Geometry: final body of the model. Coordinates: model frame, mm. Face numbers are marked on the shaded views. A direction names the side the tool comes from. Give positions to 0.01 mm unless a question says otherwise; leave off trailing zeros. Write each loop counter-clockwise with the first axis right and the second up, starting at its lowest first coordinate (ties: lowest second). Pieces come first, ordered by that corner, then holes.
Q1. Pin query (flat end, axial travel): pin 1 (6 mm diameter, centred on x = -40, z = -29.5, fed in from +Y); pin 2 (10 mm diameter, centred on y = 5.5, z = 18.5, fed in from -X) (3 decimals); pin 3 (1 mm diameter, centred on x = 4, y = 25.5, fed in from -Z) (3 decimals). Return the tip coordinate at first contact, or that it passes through.
Q2. Reachability of the marked faces 1 and 2 from +Z, -Z, +X, -X, +Y, -Y: full face, straight path, thin tool, end or side. Return the list, or none.
Q3. Cut plane D-D on x = -46. Return the cut outline in (y, z) (3 decimals), plus the area to 3 significant figures.
Q4. Line query: L1, parallel to Z at x = -40, y = 29 (3 decimals); L2, parallel to X at y = 29.35, z = 0 (3 decimals); L3, parallel to Z at x = 0, y = 28.35 (3 decimals). Output: solid intervals per line, ascending.
Q5. Cut plane A-A on y = 20.5. Return the cut outline in (x, z) (3 decimals).
Q6. Draft query along Z for the marked faces 3, 4 and 5. Return one class per face: pulls with the +Z half, pulls with the -Z half, needs draft (parallel to the pull), parting line crosses it, or undercut.
Autodesk Inventor part; units mm, degrees
ref_plane "YZ Plane" through (0, 0, 0) normal (1, 0, 0) x (0, 1, 0)
ref_plane "XZ Plane" through (0, 0, 0) normal (0, 1, 0) x (-1, 0, 0)
ref_plane "XY Plane" through (0, 0, 0) normal (0, 0, 1) x (1, 0, 0)
sketch "스케치2" plane through (0, 0, 0) normal (0, 1, 0) x (-1, 0, 0)
  line L0 (-49.375, 35.275) -> (49.375, 35.275)
  line L1 (49.375, 35.275) -> (49.375, -35.275)
  line L2 (49.375, -35.275) -> (-49.375, -35.275)
  line L3 (-49.375, -35.275) -> (-49.375, 35.275)
  line L4 (-49.375, 35.275) -> (49.375, -35.275) construction
  line L5 (49.375, 35.275) -> (-49.375, -35.275) construction
  line L6 (-54.375, -40.275) -> (54.375, -40.275)
  line L7 (54.375, -40.275) -> (54.375, 40.275)
  line L8 (54.375, 40.275) -> (-54.375, 40.275)
  line L9 (-54.375, 40.275) -> (-54.375, -40.275)
  point P0 (0, 0)
  dimension "d0" = 98.75
  dimension "d1" = 70.55
  dimension "d2" = 5
extrude "돌출1" add sketch "스케치2" along normal blind 32
sketch "스케치3" plane through (0, 0, 0) normal (0, 1, 0) x (-1, 0, 0)
  line L0 (-54.375, 40.275) -> (-54.375, -40.275) construction
  line L1 (54.375, -40.275) -> (-54.375, -40.275)
  line L2 (-54.375, -40.275) -> (-54.375, 40.275)
  line L3 (-54.375, 40.275) -> (54.375, 40.275)
  line L4 (54.375, 40.275) -> (54.375, -40.275)
  line L5 (54.375, -40.275) -> (-54.375, 40.275) construction
  line L6 (-54.375, -40.275) -> (54.375, 40.275) construction
  point P0 (0, 0)
extrude "돌출2" add sketch "스케치3" against normal blind 5
sketch "스케치4" plane through (0, 0, 0) normal (0, 1, 0) x (-1, 0, 0)
  line L0 (49.375, 35.275) -> (49.375, -35.275) construction
  line L1 (54.375, -40.275) -> (54.375, 40.275) construction
  line L2 (49.375, 30.275) -> (54.375, 30.275)
  line L3 (54.375, 30.275) -> (54.375, -30.275)
  line L4 (54.375, -30.275) -> (49.375, -30.275)
  line L5 (49.375, -30.275) -> (49.375, 30.275)
  line L6 (-49.375, 35.275) -> (49.375, 35.275) construction
  line L7 (49.375, -35.275) -> (-49.375, -35.275) construction
  line L8 (54.375, -40.275) -> (-54.375, -40.275) construction
  line L9 (-44.375, -35.275) -> (14.375, -35.275)
  line L10 (14.375, -35.275) -> (14.375, -40.275)
  line L11 (14.375, -40.275) -> (-44.375, -40.275)
  line L12 (-44.375, -40.275) -> (-44.375, -35.275)
  line L13 (-49.375, -35.275) -> (-49.375, 35.275) construction
  point P0 (0, 0)
  dimension "d7" = 5
  dimension "d8" = 5
  dimension "d11" = 5
  dimension "d12" = 35
extrude "돌출3" cut sketch "스케치4" along normal through all
sketch "스케치5" plane through (0, 32, 0) normal (0, 1, 0) x (1, 0, 0)
  line L0 (49.375, 35.275) -> (49.375, -35.275) construction
  line L1 (49.375, -35.275) -> (-49.375, -35.275) construction
  circle A0 centre (0, -37.775) radius 1.5
  circle A1 centre (51.875, 0) radius 1.5
  circle A2 centre (-34.375, 37.775) radius 1.5
  line L2 (-49.375, 35.275) -> (-14.375, 35.275) construction
  line L3 (-54.375, 40.275) -> (-54.375, 30.275) construction
  point P0 (0, 0)
  dimension "d17" = 3
  dimension "d18" = 2.5
  dimension "d19" = 3
  dimension "d20" = 2.5
  dimension "d21" = 3
  dimension "d22" = 2.5
  dimension "d23" = 20
extrude "돌출4" cut sketch "스케치5" against normal blind 5
fillet "모깎기1" radius 2.5 14 edges at (-54.375, 13.5, 40.275) (54.375, 13.5, 40.275) (54.375, 13.5, -40.275) (-54.375, 13.5, -40.275) (-54.375, -5, 0) (0, -5, -40.275) (0, -5, 40.275) (54.375, -5, 0) (-14.375, 16, -40.275) (15, 0, -40.275) (44.375, 16, -40.275) (-54.375, 16, 30.275) (-54.375, 0, 0) (-54.375, 16, -30.275)
chamfer "모따기1" distance 2 angle 45 6 edges at (-31.875, 32, -35.275) (-49.375, 32, -32.775) (-49.375, 32, 32.775) (0, 32, 35.275) (49.375, 32, 0) (46.875, 32, -35.275)
properties part number "housing_bottom"
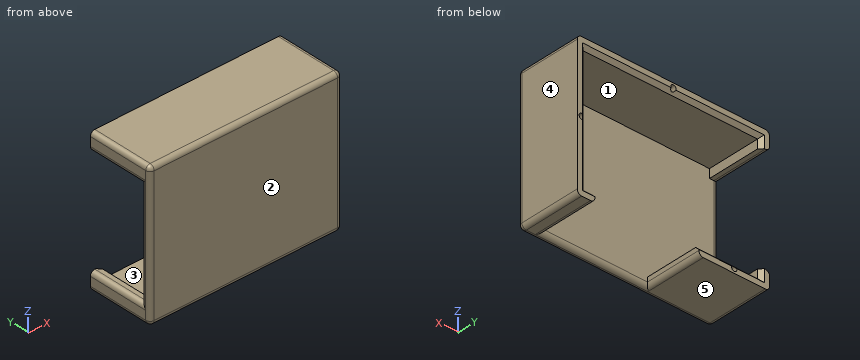
Data:
1. pin 1: stops at y = 0
1. pin 2: stops at x = 49.375
1. pin 3: stops at z = 35.275
2. face 1: +Y
2. face 2: +Z, -Z, +X, -X, -Y
3. outline: (-5, -37.775) arc R2.5 ccw to (-2.5, -40.275) - (32, -40.275) - (32, -37.275) - (30, -35.275) - (0, -35.275) - (0, 35.275) - (30, 35.275) - (32, 37.275) - (32, 40.275) - (-2.5, 40.275) arc R2.5 ccw to (-5, 37.775) - close
3. area: 716 mm2
4. L1: z = -40.275 to -35.275, 35.275 to 40.275
4. L2: x = 49.375 to 50.375, 53.375 to 54.375
4. L3: z = 35.275 to 36.275, 39.275 to 40.275
5. outline: (-54.375, -37.775) arc R2.5 ccw to (-51.875, -40.275) - (-16.875, -40.275) arc R2.5 ccw to (-14.375, -37.775) - (-14.375, -35.275) - (-49.375, -35.275) - (-49.375, -30.275) - (-51.875, -30.275) arc R2.5 ccw to (-54.375, -32.775) - close; (-54.375, 32.775) arc R2.5 ccw to (-51.875, 30.275) - (-49.375, 30.275) - (-49.375, 35.275) - (49.375, 35.275) - (49.375, -35.275) - (44.375, -35.275) - (44.375, -37.775) arc R2.5 ccw to (46.875, -40.275) - (51.875, -40.275) arc R2.5 ccw to (54.375, -37.775) - (54.375, 37.775) arc R2.5 ccw to (51.875, 40.275) - (-51.875, 40.275) arc R2.5 ccw to (-54.375, 37.775) - close
6. face 3: undercut
6. face 4: needs draft
6. face 5: pulls with the -Z half
